Input: part model. Units: mm. Frame: model coordinates. Round coordinates to 2 decimals unless told otherwise and drop trailing zeros. Write each loop counter-clockwise with the first axis right and the second up, starting at its lowest first coordinate (ties: lowest second). Pieces come first, ordered by that corner, then holes. Notation, with made-up numbers: (-33.5, -19) - (-13.5, -19) arc R24 cw to (-13.5, 7) - close; hole circle Ø5 at (-24, 3). An arc over 180 degrees is marked (long way). Use one line per item in the form item = value.
```python
from build123d import *

# Parameters (mm, degrees)
BOSS_EXTRUDE1_DEPTH = 101.6
FILLET1_R           = 0.254
SKETCH3_W           = 73.152
SKETCH3_H           = 98.552
BOSS_EXTRUDE2_DEPTH = 0.254
SKETCH4_W           = 75.692
SKETCH4_H           = 101.092
BOSS_EXTRUDE3_DEPTH = 0.635
SKETCH5_W           = 5.245580378
SKETCH5_H           = 8.524068114
SKETCH5_H_2         = 8.524068115
SKETCH5_W_2         = 5.245580379
BOSS_EXTRUDE4_DEPTH = 0.635


with BuildPart() as part:
    # Sketch1 → Boss-Extrude1 (new body)
    with BuildSketch(Plane(origin=(0, 0, 0), x_dir=(1, 0, 0), z_dir=(0, 1, 0))):
        Polygon((0, 0), (76.2, 0), (76.2, 3.81), (0, 1.1764495), align=None)
    extrude(amount=BOSS_EXTRUDE1_DEPTH)

    # Fillet1
    fillet1_edges = [part.edges().sort_by_distance(p)[0] for p in [
        (76.2, 101.6, -1.905),
        (38.1, 101.6, -2.49322475),
        (0, 101.6, -0.58822475),
        (38.1, 0, -2.49322475),
        (38.1, 0, 0),
        (0, 0, -0.58822475),
        (38.1, 101.6, 0),
        (0, 50.8, -1.1764495),
        (76.2, 50.8, -3.81),
        (76.2, 50.8, 0),
        (0, 50.8, 0),
    ]]
    fillet(fillet1_edges, radius=FILLET1_R)

    # Sketch3 → Boss-Extrude2 (add)
    with BuildSketch(Plane.XY):
        with Locations((38.1, 50.8)):
            Rectangle(SKETCH3_W, SKETCH3_H)
    extrude(amount=BOSS_EXTRUDE2_DEPTH)

    # Sketch4 → Boss-Extrude3 (add)
    with BuildSketch(Plane.XY.offset(0.254)):
        with Locations((38.1, 50.8)):
            Rectangle(SKETCH4_W, SKETCH4_H)
    extrude(amount=BOSS_EXTRUDE3_DEPTH)

    # Sketch5 → Boss-Extrude4 (add)
    with BuildSketch(Plane(origin=(-0.040610799, 0, -1.175045949), x_dir=(-0.9994033020943162, 0, 0.034540407684001274), z_dir=(-0.034540407684001274, 0, -0.9994033020943162))):
        with Locations((-3.874536836, 96.295602006)):
            Rectangle(SKETCH5_W, SKETCH5_H)
        with Locations((-71.552678444, 95.59737493)):
            Rectangle(SKETCH5_W, SKETCH5_H_2)
        with Locations((-71.735567304, 5.801534056)):
            Rectangle(SKETCH5_W, SKETCH5_H_2)
        with Locations((-4.423527668, 5.776498119)):
            Rectangle(SKETCH5_W_2, SKETCH5_H)
    extrude(amount=BOSS_EXTRUDE4_DEPTH)


solid = part.part
```
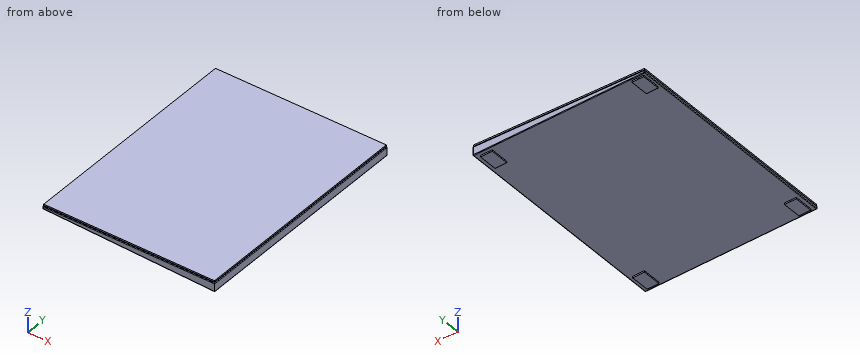
(1) Material intervals for L1, parallel to Z at x = 68.5, y = 30.5; L2, parallel to X at y = 68.5, z = -0.2; L3, parallel to Y at x = 29.5, z = 0.35, sorted ascending.
Derived:
L1 = -3.54 to 0.89
L2 = 0.01 to 76.19
L3 = 0.25 to 101.35
(2) Cut plane A-A on y = 23.5. Output: boundary loops of the cut face in (x, z), then the cut area to 3 significant figures.
Derived:
outline = (0, -0.93) arc R0.25 ccw to (0.25, -1.18) - (75.94, -3.8) arc R0.25 ccw to (76.2, -3.55) - (76.2, -0.25) arc R0.25 ccw to (75.95, 0) - (74.68, 0) - (74.68, 0.25) - (75.95, 0.25) - (75.95, 0.89) - (0.25, 0.89) - (0.25, 0.25) - (1.52, 0.25) - (1.52, 0) - (0.25, 0) arc R0.25 ccw to (0, -0.25) - close
area = 257 mm^2
(3) First-contact query: pin 1 Ø0.5 at (y, z) = (46, 0.5) entering from -X; pin 2 Ø0.7 at (x, z) = (44.5, 0.5) entering from +Y; pin 3 Ø12 at (x, y) = (57.5, 12.5) entering from -Z. Flat tips, straight axial feed; report the tip coordinate or a pass-through.
Derived:
pin_1 = 0.25
pin_2 = 101.35
pin_3 = -3.37
